Part model, mm, in its own coordinate system. A direction names the side the tool comes from. Coordinates: 2 decimals unless noted, no trailing zeros. Order: outer loops, then holes, each group sorted by start corner. A loop starts at its lowest first (then second) coordinate and runs counter-clockwise, first axis right, second up. Notation, with made-up numbers: (74, 3) - (89, 3) arc R18 cw to (89, 18) - close; hole circle Ø6 at (86, 22). An arc over 180 degrees is marked (long way). Use a Markdown table: item, result. Add a question column.
1) Saw through at A-A on y = -6. List the corners of the cut face in (x, z), then the cut area to 3 significant figures.
2) Two-plate mould, pull along Z, no slides. Class faces 3 (the face through (7, -13, 6.35)), 4 (the face through (74, -31.75, 6)), 5 (the face through (9.08, -12.52, 18.87)), 6 (the face through (7.287, -12.522, -19.046)): +Z half, -Z half, draft (parallel to the pull), parting line (faces both ways), or undercut.
3) Tool access for faces 1 (the face through (-24.25, -12.52, -0.14)), 2 (the face through (-55, -38.1, 19)): list every direction of +Z, -Z, +X, -X, +Y, -Y with a clear straight run to the whole face (end or side of a thin tool).
4) Drop flat-ended pins along their axis: P1, Ø20.5, axis at x = 1.5, y = -8, coming from the +Z side; P2, Ø8, axis at x = 66.5, y = -28, coming from the +Z side; P3, Ø12.5, axis at x = 11, y = -7.5, coming from the -Z side; P4, Ø23, axis at x = -58.37, z = 0, coming from the -Y side. Give the stop position or say it passes through.
5) Saw through at C-C on x = -10.5. List the corners of the cut face in (y, z), then the cut area to 3 significant figures.
6) Saw through at B-B on x = -59. List the corners of the cut face in (y, z), then the cut area to 3 significant figures.
7) Saw through at D-D on z = -20.5. List the corners of the cut face in (x, y), then the cut area to 3 significant figures.
8) Wall check: L1, parallel to X at y = -19.5, z = 3.5; L2, parallel to Y at x = -41, z = 21; L3, parallel to Z at x = -60, y = -5.5. Give the ranges that are in metal, low to high. Write a range as [from, to].
```python
from build123d import *

# Parameters (mm, degrees)
F0_R     = 19.05
F1_DEPTH = 38.1
F2_DEPTH = 25.4
F0_R_2   = 6.35
F3_DEPTH = 31.75


with BuildPart() as f1:
    # F0 (on Front) → F1 (new body)
    with BuildSketch(Plane.XZ):
        with BuildLine():
            ThreePointArc((-55.877387, -25.277314), (-39.549404, -17.05617), (-32.970856, 0))
            ThreePointArc((-32.970856, 0), (-39.549404, 17.05617), (-55.877387, 25.277314))
            ThreePointArc((-55.877387, 25.277314), (-83.770856, 0), (-55.877387, -25.277314))
        make_face()
        with Locations((-58.370856, 0)):
            Circle(F0_R, mode=Mode.SUBTRACT)
    extrude(amount=F1_DEPTH)

    # F0 (on Front) → F2 (join)
    with BuildSketch(Plane.XZ):
        with BuildLine():
            ThreePointArc((-55.877387, 25.277314), (-39.549404, 17.05617), (-32.970856, 0))
            ThreePointArc((-32.970856, 0), (-39.549404, -17.05617), (-55.877387, -25.277314))
            Line((-55.877387, -25.277314), (72.245812, -12.638657))
            ThreePointArc((72.245812, -12.638657), (58.299077, 0), (72.245812, 12.638657))
            Line((72.245812, 12.638657), (-55.877387, 25.277314))
        make_face()
        with BuildLine():
            ThreePointArc((-17.900923, -6.35), (-24.250923, 0), (-17.900923, 6.35))
            Line((-17.900923, 6.35), (32.899077, 6.35))
            ThreePointArc((32.899077, 6.35), (37.389205, 4.490128), (39.249077, 0))
            ThreePointArc((39.249077, 0), (37.389205, -4.490128), (32.899077, -6.35))
            Line((32.899077, -6.35), (-17.900923, -6.35))
        make_face(mode=Mode.SUBTRACT)
    extrude(amount=F2_DEPTH)

    # F0 (on Front) → F3 (join)
    with BuildSketch(Plane.XZ):
        with BuildLine():
            ThreePointArc((83.699077, 0), (80.409803, 8.528085), (72.245812, 12.638657))
            ThreePointArc((72.245812, 12.638657), (58.299077, 0), (72.245812, -12.638657))
            ThreePointArc((72.245812, -12.638657), (80.409803, -8.528085), (83.699077, 0))
        make_face()
        with Locations((70.999077, 0)):
            Circle(F0_R_2, mode=Mode.SUBTRACT)
    extrude(amount=F3_DEPTH)


solid = f1.part
```
Results are:
| question | item | result |
|---|---|---|
| 1 | outline | (-55.88, -25.28) - (72.25, -12.64) arc R12.7 ccw to (72.25, 12.64) - (-55.88, 25.28) arc R25.4 ccw (long way) to start; hole circle Ø38.1 at (-58.37, 0); hole (-17.9, -6.35) - (32.9, -6.35) arc R6.35 ccw to (32.9, 6.35) - (-17.9, 6.35) arc R6.35 ccw to start; hole circle Ø12.7 at (71, 0) |
| 1 | area | 4,180 mm2 |
| 2 | face 3 | undercut |
| 2 | face 4 | draft |
| 2 | face 5 | +Z half |
| 2 | face 6 | -Z half |
| 3 | face 1 | +Y, -Y |
| 3 | face 2 | +Z, -Z, +X, -X, -Y |
| 4 | P1 | z = 20.63 |
| 4 | P2 | z = 13.51 |
| 4 | P3 | z = -19.3 |
| 4 | P4 | through |
| 5 | outline | (-25.4, -20.8) - (0, -20.8) - (0, -6.35) - (-25.4, -6.35) - close; (-25.4, 6.35) - (0, 6.35) - (0, 20.8) - (-25.4, 20.8) - close |
| 5 | area | 734 mm2 |
| 6 | outline | (-38.1, -25.39) - (0, -25.39) - (0, -19.04) - (-38.1, -19.04) - close; (-38.1, 19.04) - (0, 19.04) - (0, 25.39) - (-38.1, 25.39) - close |
| 6 | area | 484 mm2 |
| 7 | outline | (-73.37, -38.1) - (-43.37, -38.1) - (-43.37, -25.4) - (-7.45, -25.4) - (-7.45, 0) - (-73.37, 0) - close |
| 7 | area | 2,060 mm2 |
| 8 | L1 | [-83.53, -77.1], [-39.65, -23.2], [38.2, 65.7], [76.3, 83.21] |
| 8 | L2 | [-25.4, 0] |
| 8 | L3 | [-25.35, -18.98], [18.98, 25.35] |
